```python
from build123d import *

# Parameters (mm, degrees)
SKETCH2_R = 0.7366


with BuildPart() as part:
    # Sweep1: sweep along a path in Sketch1
    with BuildLine(Plane(origin=(0, 0, 0), x_dir=(0, 0, -1), z_dir=(1, 0, 0))) as sweep1_path:
        Line((-42.483763873, -0.7366), (-39.364266321, -0.7366))
        ThreePointArc((-39.364266321, -0.7366), (-38.913706182, -0.746755379), (-38.464061165, -0.777200888))
        Line((-38.464061165, -0.777200888), (-0.381380916, -4.219399028))
        ThreePointArc((-0.381380916, -4.219399028), (4.2366, 0), (-0.381380916, 4.219399028))
        Line((-0.381380916, 4.219399028), (-38.464061165, 0.777200888))
        ThreePointArc((-38.464061165, 0.777200888), (-38.913706182, 0.746755379), (-39.364266321, 0.7366))
        Line((-39.364266321, 0.7366), (-42.483763873, 0.7366))
        Line((-42.483763873, 0.7366), (-54.56460022, 0.7366))
    # Sketch2 → Sweep1 (sweep)
    with BuildSketch(Plane.XY.offset(54.56460022)):
        with Locations((0, 0.7366)):
            Circle(SKETCH2_R)
    sweep(path=sweep1_path.line)


solid = part.part
```
Design review of the part built by this model. Coordinates are the model's own, in mm. Round coordinates to 2 decimals unless told otherwise and drop trailing zeros. Write each loop counter-clockwise with the first axis right and the second up, starting at its lowest first coordinate (ties: lowest second). Pieces come first, ordered by that corner, then holes.
Item 1: We need section B-B on x = -0.4. Write out the cut boundary in (y, z).
Item 2: For probe 1 along Y at (x, z) = (0.3, 24); probe 2 along Y at (x, z) = (0.55, 11); probe 3 along Y at (x, z) = (0.15, 49.5), list the stretches that pass through material, from the lowest coordinate up.
Item 3: We need section A-A on z = 43. Write out the cut boundary in (x, y), and give its area (3 significant figures).
Item 4: The part is to be moulded in two halves that separate along Z. For faces 1 (the flat face through (0, -1, 42.484)), 2 (the cylindrical face through (0.4, 3.09, 19.75)), say which applies: +Z half, -Z half, draft (parallel to the pull), parting line (faces both ways), or undercut.
Returned:
1. outline: (-4.84, 0.44) arc R4.86 ccw (long way) to (4.84, 0.44) - (1.39, 38.52) arc R9.38 cw to (1.36, 39.36) - (1.36, 54.56) - (0.12, 54.56) - (0.12, 39.36) arc R10.62 ccw to (0.16, 38.41) - (3.6, 0.33) arc R3.62 cw (long way) to (-3.6, 0.33) - (-0.16, 38.41) arc R10.62 ccw to (-0.12, 39.36) - (-0.12, 42.48) - (-1.36, 42.48) - (-1.36, 39.36) arc R9.38 cw to (-1.39, 38.52) - close
2. probe 1: y = -2.76 to -1.41, 1.41 to 2.76
2. probe 2: y = -3.75 to -2.77, 2.77 to 3.75
2. probe 3: y = 0.02 to 1.46
3. outline: circle Ø1.47 at (0, 0.74)
3. area: 1.70 mm2
4. face 1: +Z half
4. face 2: undercut
